from build123d import *

# Parameters (mm, degrees)
SKETCH1_W           = 19.05
SKETCH1_H           = 38.1
SKETCH1_W_2         = 12.7
SKETCH1_H_2         = 31.75
BOSS_EXTRUDE1_DEPTH = 50.8
SKETCH2_R           = 3.175
CUT_EXTRUDE1_DEPTH  = 20.05
CUT_EXTRUDE2_REACH  = 21.05
SKETCH3_R           = 4.7625
SKETCH4_R           = 2.667
CUT_EXTRUDE3_DEPTH  = 20.05
CUT_EXTRUDE4_REACH  = 21.05
SKETCH5_R           = 4.7625


with BuildPart() as part:
    # Sketch1 → Boss-Extrude1 (new body)
    with BuildSketch(Plane(origin=(0, 0, 0), x_dir=(1, 0, 0), z_dir=(0, 1, 0))):
        with Locations((9.525, 19.05)):
            Rectangle(SKETCH1_W, SKETCH1_H)
        with Locations((9.525, 19.05)):
            Rectangle(SKETCH1_W_2, SKETCH1_H_2, mode=Mode.SUBTRACT)
    extrude(amount=BOSS_EXTRUDE1_DEPTH)

    # Sketch2 → Cut-Extrude1 (cut, through all)
    with BuildSketch(Plane(origin=(19.05, 0, 0), x_dir=(0, 0, -1), z_dir=(1, 0, 0))):
        with Locations((19.05, 15.40002)):
            Circle(SKETCH2_R)
        with Locations((19.05, 35.39998)):
            Circle(SKETCH2_R)
    extrude(amount=-CUT_EXTRUDE1_DEPTH, mode=Mode.SUBTRACT)

    # Sketch3 → Cut-Extrude2 (cut, up to next)
    with BuildSketch(Plane(origin=(19.05, 0, 0), x_dir=(0, 0, -1), z_dir=(1, 0, 0)), mode=Mode.PRIVATE) as cut_extrude2_sk1:
        with Locations((19.05, 15.40002)):
            Circle(SKETCH3_R)
    cut_extrude2_tool1 = extrude(cut_extrude2_sk1.sketch, amount=-CUT_EXTRUDE2_REACH, mode=Mode.PRIVATE) & part.part
    add(cut_extrude2_tool1.solids().sort_by_distance((19.05, 15.40002, -19.05))[0], mode=Mode.SUBTRACT)
    # Sketch3 → Cut-Extrude2 (cut, up to next)
    with BuildSketch(Plane(origin=(19.05, 0, 0), x_dir=(0, 0, -1), z_dir=(1, 0, 0)), mode=Mode.PRIVATE) as cut_extrude2_sk2:
        with Locations((19.05, 35.39998)):
            Circle(SKETCH3_R)
    cut_extrude2_tool2 = extrude(cut_extrude2_sk2.sketch, amount=-CUT_EXTRUDE2_REACH, mode=Mode.PRIVATE) & part.part
    add(cut_extrude2_tool2.solids().sort_by_distance((19.05, 35.39998, -19.05))[0], mode=Mode.SUBTRACT)

    # Sketch4 → Cut-Extrude3 (cut, through all)
    with BuildSketch(Plane.ZY):
        with Locations((-19.05, 25.4)):
            Circle(SKETCH4_R)
    extrude(amount=-CUT_EXTRUDE3_DEPTH, mode=Mode.SUBTRACT)

    # Sketch5 → Cut-Extrude4 (cut, up to next)
    with BuildSketch(Plane.ZY, mode=Mode.PRIVATE) as cut_extrude4_sk1:
        with Locations((-19.05, 25.4)):
            Circle(SKETCH5_R)
    cut_extrude4_tool1 = extrude(cut_extrude4_sk1.sketch, amount=-CUT_EXTRUDE4_REACH, mode=Mode.PRIVATE) & part.part
    add(cut_extrude4_tool1.solids().sort_by_distance((0, 25.4, -19.05))[0], mode=Mode.SUBTRACT)


solid = part.part
The model under review builds one solid part; all positions refer to its coordinate system, in mm. A direction names the side the tool comes from. Coordinates: 2 decimals unless noted, no trailing zeros. Write each loop counter-clockwise with the first axis right and the second up, starting at its lowest first coordinate (ties: lowest second). Pieces come first, ordered by that corner, then holes. Notation, with made-up numbers: (74.25, 19.25) - (110.25, 19.25) arc R20 cw to (110.25, 47.25) - close; hole circle Ø11 at (-14, 40). An arc over 180 degrees is marked (long way). Answer as a JSON object with one key per item and string values. Group by question number.
1. Add section C-C (y = 3). Give the boundary of the cut face in (x, z) (3 decimals).
2. Add section B-B (x = 8.75). Give the boundary of the cut face in (y, z) (3 decimals), plus the area to 3 significant figures.
3. Machinability: for faces 1 (the face through (17.48, 12.5, -15.27)), 2 (the face through (1.6, 26.8, -14.5)), 3 (the face through (3.175, 31, -19)), 4 (the face through (3, 0, -19)), which of the approach directions +Z, -Z, +X, -X, +Y, -Y give a long, thin tool a straight path to every point of the face, cutting with its end or side? Answer none if there is none.
4. To check wall thickness, follow probe 1 along Y at (x, z) = (2.05, -19.05); probe 2 along Y at (x, z) = (17.35, -19.05); probe 3 along Z at (x, y) = (6.25, 18) (3 decimals). State the ranges of each line that lie inside material, in increasing order.
5. Mouldability with a two-part tool opening along Z and no side actions: class faces 5 (the face through (9, 25, -38.1)), 6 (the face through (19.05, 25, -15)), 7 (the face through (17.485, 35.609, -14.292)) as pulls with the +Z half, pulls with the -Z half, needs draft (parallel to the pull), parting line crosses it, or undercut.
6. Clearance check with a flat-ended pin moving along its axis: pin 1 Ø5 at (y, z) = (35.4, -19.05) entering from +X. State where the tip first meets the part, or that it passes through.
7. Add section A-A (z = -19.05). Give the number of separate pieces and of enclosed holes in the cut face, plus the area to 3 significant figures.
Findings:
{
 "1": {"outline": "(0, -38.1) - (19.05, -38.1) - (19.05, 0) - (0, 0) - close; hole (3.175, -34.925) - (15.875, -34.925) - (15.875, -3.175) - (3.175, -3.175) - close"},
 "2": {"outline": "(0, -38.1) - (50.8, -38.1) - (50.8, -34.925) - (0, -34.925) - close; (0, -3.175) - (50.8, -3.175) - (50.8, 0) - (0, 0) - close", "area": "323 mm²"},
 "3": {"face 1": "+X", "face 2": "-X", "face 3": "+Y, -Y", "face 4": "+Z, -Z, +X, -X, -Y"},
 "4": {"probe 1": "0 to 12.23, 18.58 to 20.64, 30.16 to 32.22, 38.57 to 50.8", "probe 2": "0 to 10.64, 20.16 to 22.73, 28.07 to 30.64, 40.16 to 50.8", "probe 3": "-38.1 to -34.925, -3.175 to 0"},
 "5": {"face 5": "pulls with the -Z half", "face 6": "needs draft", "face 7": "undercut"},
 "6": {"pin 1": "through"},
 "7": {"separate pieces": "8", "enclosed holes": "0", "area": "175 mm²"}
}
